from build123d import *

# Parameters (mm, degrees)
BASENUT_START = -5.2
BASENUTSKE_R  = 2.5
BASENUT_DEPTH = 5.2
SKETCH4_W     = 0.5
SKETCH4_H     = 10.773502692


# Read off the part's stored shape, not the designer's step: ThreadSchematic
with BuildPart() as part:
    # BaseNutSke → BaseNut (new body)
    with BuildSketch(Plane.XY.offset(BASENUT_START)):
        Polygon((5, 2.886751346), (5, -2.886751346), (0, -5.773502692), (-5, -2.886751346), (-5, 2.886751346), (0, 5.773502692), align=None)
        Circle(BASENUTSKE_R, mode=Mode.SUBTRACT)
    extrude(amount=BASENUT_DEPTH)

    # Sketch5 (on Front Plane) → EndChamfer (revolve, cut)
    with BuildSketch(Plane.XY):
        Polygon((5.1746, 3), (4.789485854, 2.45), (5.2254, 2.45), (5.2254, 3), align=None)
    revolve(axis=Axis((5.2254, 2.45, 0), (-1, 0, 0)), mode=Mode.SUBTRACT)

    # Sketch4 → Bearing-Face (revolve, cut)
    with BuildSketch(Plane(origin=(0, 0, 0), x_dir=(0, 0, -1), z_dir=(1, 0, 0)), mode=Mode.PRIVATE) as bearing_face_sk:
        with Locations((4.95, 10.386751346)):
            Rectangle(SKETCH4_W, SKETCH4_H)
        Polygon((0, 5), (-10, 5), (-10, 15.773502692), (0.446581987, 15.773502692), (0.446581987, 5.773502692), align=None)
    revolve(bearing_face_sk.sketch.rotate(Axis((0, 0, 0), (0, 0, -1)), 90), axis=Axis((0, 0, 0), (0, 0, -1)), mode=Mode.SUBTRACT)

    # ThreadSchematic outline → ThreadSchematic (revolve, cut)
    with BuildSketch(Plane.XZ):
        Polygon((2.5, 0), (2.5, -0.350103769), (3, 0), align=None)
        Polygon((3, -5.1746), (2.5, -4.824496231), (2.5, -5.2), (3, -5.2), align=None)
    revolve(axis=Axis((0, 0, 0), (0, 0, 1)), mode=Mode.SUBTRACT)


solid = part.part
Here's how the part is built. I have some questions about the finished solid (model axes, mm). A direction names the side the tool comes from. Coordinates: 2 decimals unless noted, no trailing zeros. Write each loop counter-clockwise with the first axis right and the second up, starting at its lowest first coordinate (ties: lowest second). Pieces come first, ordered by that corner, then holes.
1) Which directions (+Z, -Z, +X, -X, +Y, -Y) give clear straight access to the entire face, cutting with the end or side of a thin tool? Please do faces 1 (the face through (4.5, -2.7, -4.7)), 2 (the face through (4.5, 2.6, -4.7)), 3 (the face through (-4.5, 2.6, -4.7)).
Filled in:
face 1: -Z, +X, -Y
face 2: -Z, +X, +Y
face 3: -Z, -X, +Y
2) If we section it at A-A (z = -2): List the corners of the cut face in (x, y) for me, plus the area to 3 significant figures.
Filled in:
outline: (-5, -2.89) - (0, -5.77) - (5, -2.89) - (5, 2.89) - (0, 5.77) - (-5, 2.89) - close; hole circle Ø5 at (0, 0)
area: 67.0 mm2
3) Thinking about a two-plate mould opening in X: for faces 4 (the face through (-4.5, -2.7, -4.7)), 5 (the face through (-0.54, -2.44, -2.62)), 6 (the face through (2.535, -4.31, -2.383)), which applies, +X half, -X half, draft (parallel to the pull), parting line (faces both ways), or undercut?
Filled in:
face 4: draft
face 5: undercut
face 6: +X half
4) If I drill on line 1 (Y direction, x = 1.5, z = -1.4); line 2 (Y direction, x = 0, z = -5.15); line 3 (X direction, y = 1.5, z = -0.5), over which ranges is the centre line in solid material (lowest first)?
Filled in:
line 1: y = -4.91 to -2, 2 to 4.91
line 2: y = -5 to -2.96, 2.96 to 5
line 3: x = -5 to -2, 2 to 5
